Part model, mm, in its own coordinate system. Give positions to 0.01 mm unless a question says otherwise; leave off trailing zeros. Write each loop counter-clockwise with the first axis right and the second up, starting at its lowest first coordinate (ties: lowest second). Pieces come first, ordered by that corner, then holes. Notation, with made-up numbers: M 14.25,-24.75 L 61.25,-24.75 A17 cw 61.25,-18.75 Z; hole C -37,11.5 d2. An arc over 180 degrees is marked long. Write item = value, one per line. Start each with the question number.
Autodesk Inventor part; units mm, degrees
ref_plane "YZ Plane" through (0, 0, 0) normal (1, 0, 0) x (0, 1, 0)
ref_plane "XZ Plane" through (0, 0, 0) normal (0, 1, 0) x (-1, 0, 0)
ref_plane "XY Plane" through (0, 0, 0) normal (0, 0, 1) x (1, 0, 0)
sketch "Sketch1" plane through (0, 0, 0) normal (1, 0, 0) x (0, 1, 0)
  arc A0 (18.5, 35) -> (1.5, 35) centre (10, 35) ccw
  arc A1 (1.5, 8) -> (18.5, 8) centre (10, 8) ccw
  arc A2 (23, 35) -> (-3, 35) centre (10, 35) ccw
  arc A3 (-3, 8) -> (23, 8) centre (10, 8) ccw
  line L0 (-3, 35) -> (-3, 8)
  line L1 (23, 35) -> (23, 8)
  circle A4 centre (10, 35) radius 8.5
  circle A5 centre (10, 8) radius 8.5
  dimension "d12" = 17
  dimension "d13" = 17
  dimension "d15" = 26
  dimension "d16" = 26
extrude "Extrusion1" add sketch "Sketch1" along normal blind 10
sketch "Sketch2" plane through (10, 0, 0) normal (1, 0, 0) x (0, 0, -1)
  circle A0 centre (-35, 10) radius 8.5
  circle A1 centre (-8, 10) radius 8.5
  circle A2 centre (-8, 10) radius 8.5
  line L0 (-35, 10) -> (-35, 18.5)
  circle A3 centre (-35, 10) radius 8.5
  line L1 (-35, 10) -> (-26.5, 10) construction
  line L2 (-35, 18.5) -> (-7.677334, 18.493873)
  line L3 (-8, 10) -> (-8, 1.5)
  line L4 (-8, 10) -> (0.5, 10) construction
  line L5 (-8, 1.5) -> (-35.117933, 1.500818)
  point P0 (0, 0)
  dimension "d19" = 90
  dimension "d20" = 90
sketch "Sketch2 outline for Extrusion2" plane through (10, 0, 0) normal (1, 0, 0) x (0, 0, -1)
  arc A0 (-8, 1.5) -> (-7.677334, 18.493873) centre (-8, 10) ccw
  line L0 (-35.117933, 1.500818) -> (-8, 1.5)
  arc A1 (-35, 18.5) -> (-35.117933, 1.500818) centre (-35, 10) ccw
  line L1 (-7.677334, 18.493873) -> (-35, 18.5)
extrude "Extrusion2" cut sketch "Sketch2 outline for Extrusion2" against normal blind 5
properties part number "Sensor support"
Q1. Drop flat-ended pins along their axis: P1, Ø1.5, axis at x = 5.5, y = 19, coming from the -Z side; P2, Ø3, axis at x = 8.5, y = 19, coming from the -Z side; P3, Ø8.5, axis at y = 13, z = 23, coming from the +X side. Give the stop position or say it passes through.
Q2. Two-plate mould, pull along Z, no slides. Class faces 1 (the face through (5, 10, -5)), 2 (the face through (0, 10, 22)), 3 (the face through (5, 10, 22)): +Z half, -Z half, draft (parallel to the pull), parting line (faces both ways), or undercut.
Q3. Slice it at A-A (x = 6.5). Give the cut face in (y, z).
Q4. Slice it at B-B (y = 10). Give the cut face in (x, z), and give its area (3 significant figures).
Q5. Probe line 1 along Z through (x, y) = (4.75, 10); line 2 along Z through (x, y) = (7, 10); line 3 along Y through (x, z) = (7.5, 8). List the from-to ranges inside material, lowest first.
Q6. Slice it at D-D (x = 1). Give the cut face in (y, z), and give its area (3 significant figures).
Q7. Slice it at C-C (z = 38.5). Give the cut face in (x, y), and give its area (3 significant figures).
Working result:
q1.P1 = -2.05
q1.P2 = -2.62
q1.P3 = 5
q2.face_1 = -Z half
q2.face_2 = draft
q2.face_3 = undercut
q3.outline = M -3,8 A13 ccw 23,8 L 23,35 A13 ccw -3,35 Z; hole M 1.5,8 A8.5 ccw long 18.49,8.32 L 18.5,35 A8.5 ccw long 1.5,34.88 Z
q4.outline = M 0,-5 L 10,-5 L 10,-0.5 L 0,-0.5 Z; M 0,16.5 L 5,16.5 L 5,26.5 L 0,26.5 Z; M 0,43.5 L 10,43.5 L 10,48 L 0,48 Z
q4.area = 140 mm2
q5.line_1 = -5 to -0.5, 16.5 to 26.5, 43.5 to 48
q5.line_2 = -5 to -0.5, 43.5 to 48
q5.line_3 = -3 to 1.5, 18.5 to 23
q6.outline = M -3,8 A13 ccw 23,8 L 23,35 A13 ccw -3,35 Z; hole C 10,8 d17; hole C 10,35 d17
q6.area = 779 mm2
q7.outline = M 0,-2.52 L 10,-2.52 L 10,2.25 L 0,2.25 Z; M 0,17.75 L 10,17.75 L 10,22.52 L 0,22.52 Z
q7.area = 95.5 mm2
